Check sheet for the drawn part. Datum: minimum x, y, z corner. Units: mm. A direction names the side the tool comes from. Give positions to 0.01 mm unless a question says otherwise; leave off trailing zeros. Loops run counter-clockwise (first coordinate to the right, second up) from the corner with the lowest first, then second, coordinate; pieces in that order, holes last. Notation, with made-up numbers: (-27, -29.5) - (18, -29.5) arc R20 cw to (18, 1.5) - close; hole circle Ø10 at (7.25, 89). An arc over 180 degrees is marked (long way). Use one line per item in the form item = value.
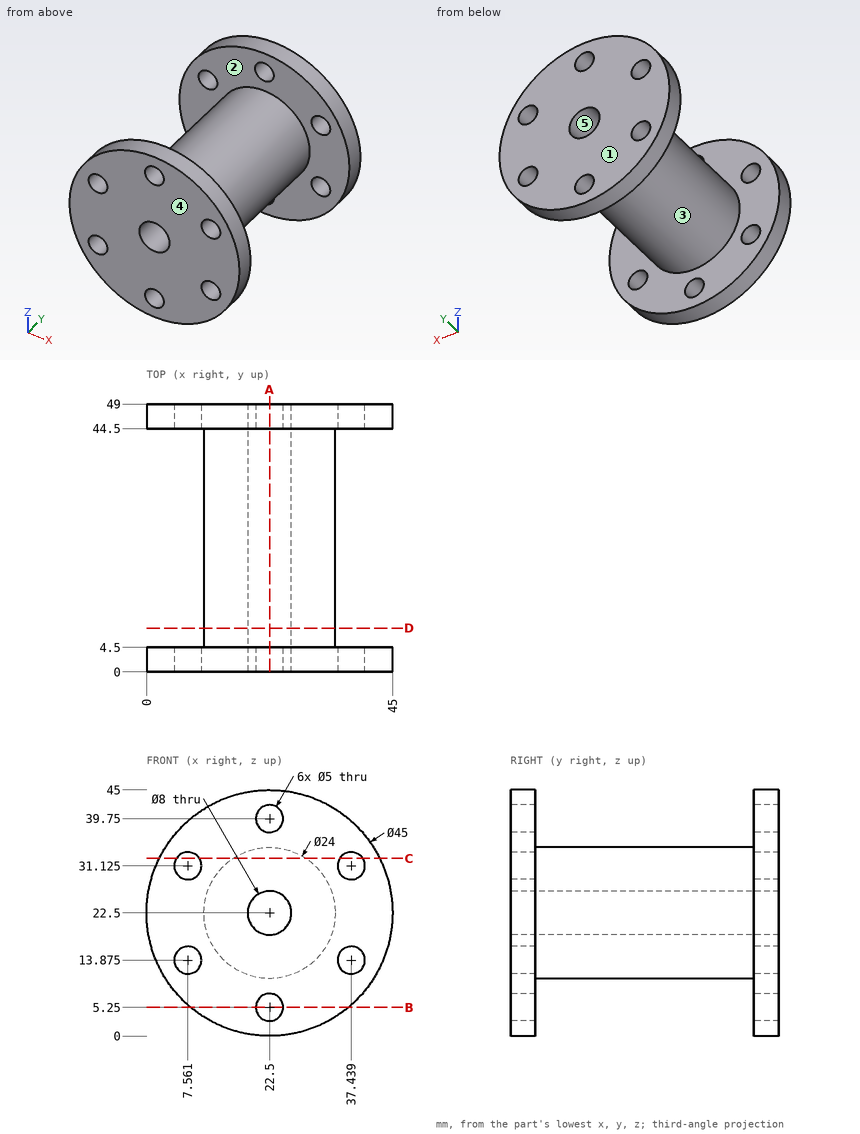
1. Section check B-B, the plane z = 5.25. Record the cut outline in (x, y), then the cut area to 3 significant figures.
Result set:
outline = (8.05, 0) - (20, 0) - (20, 4.5) - (8.05, 4.5) - close; (8.05, 44.5) - (20, 44.5) - (20, 49) - (8.05, 49) - close; (25, 0) - (36.95, 0) - (36.95, 4.5) - (25, 4.5) - close; (25, 44.5) - (36.95, 44.5) - (36.95, 49) - (25, 49) - close
area = 215 mm²
2. Depth check by flat-ended pin: pin 1 Ø2 at (x, y) = (23, 44) entering from +Z; pin 2 Ø2 at (y, z) = (39.5, 23) entering from -X; pin 3 Ø4 at (x, y) = (35.5, 7) entering from -Z. Enter the tip coordinate at first touch or a pass-through.
Result set:
pin_1 = 45
pin_2 = 10.5
pin_3 = 17.7
3. Draft check along X on the marked faces 3, 4 and 5. Enter one of: released by +X, released by -X, zero draft, split by the parting line, or undercut.
Result set:
face_3 = split by the parting line
face_4 = zero draft
face_5 = undercut
4. Tool access check on the marked faces 1 and 2. Record the directions out of +Z, -Z, +X, -X, +Y, -Y that give a thin tool (end or side, any length) a straight path to the whole face; none if there is none.
Result set:
face_1 = +Z, -Z, +X, -X, +Y
face_2 = none
5. Section check A-A, the plane x = 22.5. State how many separate pieces and enclosed holes the cut face has, then the cut area to 3 significant figures.
Result set:
separate_pieces = 6
enclosed_holes = 0
area = 883 mm²
6. Scan lines: probe 1 along Y at (x, z) = (32, 13); probe 2 along X at (y, z) = (45, 14); probe 3 along X at (y, z) = (13, 26). Record each from-to range of solid material in increasing order.
Result set:
probe_1 = 0 to 4.5, 44.5 to 49
probe_2 = 1.67 to 5.06, 10.06 to 34.94, 39.94 to 43.33
probe_3 = 11.02 to 20.56, 24.44 to 33.98
7. Section check D-D, the plane y = 8. Record the cut outline in (x, z), then the cut area to 3 significant figures.
Result set:
outline = circle Ø24 at (22.5, 22.5); hole circle Ø8 at (22.5, 22.5)
area = 402 mm²
8. Section check C-C, the plane z = 32.5. Record the cut outline in (x, y), then the cut area to 3 significant figures.
Result set:
outline = (2.34, 0) - (5.47, 0) - (5.47, 4.5) - (2.34, 4.5) - close; (2.34, 44.5) - (5.47, 44.5) - (5.47, 49) - (2.34, 49) - close; (9.65, 0) - (35.35, 0) - (35.35, 4.5) - (29.13, 4.5) - (29.13, 44.5) - (35.35, 44.5) - (35.35, 49) - (9.65, 49) - (9.65, 44.5) - (15.87, 44.5) - (15.87, 4.5) - (9.65, 4.5) - close; (39.53, 0) - (42.66, 0) - (42.66, 4.5) - (39.53, 4.5) - close; (39.53, 44.5) - (42.66, 44.5) - (42.66, 49) - (39.53, 49) - close
area = 818 mm²
